For this review, take the finished solid that the model builds, in its own axes (mm). A direction names the side the tool comes from. Coordinates: 2 decimals unless noted, no trailing zeros. Loops run counter-clockwise (first coordinate to the right, second up) from the corner with the lowest first, then second, coordinate; pieces in that order, holes last. Notation, with made-up numbers: (58, -31.5) -> (81, -31.5) arc R6 ccw to (81, -26.5) -> close; hole circle Ø3 at (37.5, -36). An arc over 180 degrees is marked (long way). Use a Markdown table: item, result.
from build123d import *

# Parameters (mm, degrees)
F1_DEPTH     = 100
F0_R         = 2
F2_DEPTH     = 3
F3_DEPTH     = 40
F4_W         = 80
F4_H         = 60
F5_DEPTH     = 2
F7_DEPTH     = 25
F9_R         = 6
F10_T1_DEPTH = 40
F10_T3_DEPTH = 47.5
F11_R        = 0.99999
F12_SIZE     = 2.2


# Not quite as in the source:
# - a fillet or chamfer that OpenCascade refuses, or shapes differently, is made with other operations: its cross-section is extruded or revolved along the edge and cut away or added
# - a fillet or chamfer is up to 0.001 mm smaller than in the source, because OpenCascade refuses the exact size


with BuildPart() as f1:
    # F0 (on Right) → F1 (new body)
    with BuildSketch(Plane.YZ):
        Polygon((34.2351660257, -7.2769091786), (0, 0), (-34.2351660257, -7.2769091786), (-33.6114309532, -10.2113519808), (0, -3.0670217846), (33.6114309532, -10.2113519808), align=None)
    extrude(amount=F1_DEPTH)

    # F0 (on Right) → F2 (join)
    with BuildSketch(Plane.YZ):
        Polygon((5.3139140418, 25), (0, 0), (34.2351660257, -7.2769091786), (63.9481604091, 132.5117388406), (29.7129943835, 139.7886480192), align=None)
        with Locations((43.711902034, 121.4779794189)):
            Circle(F0_R, mode=Mode.SUBTRACT)
        Polygon((-5.3139140418, 25), (0, 0), (5.3139140418, 25), align=None)
        Polygon((-34.2351660257, -7.2769091786), (0, 0), (-5.3139140418, 25), (-29.7129943835, 139.7886480192), (-63.9481604091, 132.5117388406), align=None)
        with Locations((-43.711902034, 121.4779794189)):
            Circle(F0_R, mode=Mode.SUBTRACT)
    extrude(amount=F2_DEPTH)

    # F0 (on Right) → F3 (join)
    with BuildSketch(Plane.YZ):
        Polygon((-33.6114309532, -10.2113519808), (-34.2351660257, -7.2769091786), (-37.1696088279, -7.9006442511), (-38.209167282, -3.0099062474), (-40.1654624834, -3.425729629), (-38.5021689569, -11.2509104349), align=None)
        Polygon((37.1696088279, -7.9006442511), (34.2351660257, -7.2769091786), (33.6114309532, -10.2113519808), (38.5021689569, -11.2509104349), (40.1654624834, -3.425729629), (38.209167282, -3.0099062474), align=None)
    extrude(amount=F3_DEPTH)

    # F4 (on face) → F5 (join)
    with BuildSketch(Plane(origin=(0, 34.2351660257, -7.2769091786), x_dir=(-1, 0, 0), z_dir=(0, 0.9781476007, -0.2079116908))):
        Polygon((-3, 106.1880215352), (-83, 60), (-3, 60), align=None)
        with Locations((-43, 30)):
            Rectangle(F4_W, F4_H)
    extrude(amount=-F5_DEPTH)

    # F6 (on face) → F7 (cut)
    with BuildSketch(Plane(origin=(0, 34.2351660257, -7.2769091786), x_dir=(-1, 0, 0), z_dir=(0, 0.9781476007, -0.2079116908))):
        Polygon((-68.2907584126, 20.9817930688), (-37.1453792063, 3), (-6, 20.9817930688), (-6, 56.9453792063), (-37.1453792063, 74.927172275), (-68.2907584126, 56.9453792063), align=None)
    extrude(amount=-F7_DEPTH, mode=Mode.SUBTRACT)

    # F8: F1 across plane


with BuildPart() as f1_1:
    add(f1.part)
    add(f1.part.mirror(Plane.XZ))

    # F9
    f9_edges = [f1_1.edges().sort_by_distance(p)[0] for p in [
        (3, -55.33475, 96.798561),
        (3, 55.33475, 96.798561),
        (83, -45.73172, 51.619859),
        (83, 45.73172, 51.619859),
        (83, -33.257018, -7.068997),
        (83, 33.257018, -7.068997),
        (1.5, -5.313914, 25),
        (1.5, 5.313914, 25),
        (51.5, 0, 0),
        (50, 0, -3.067022),
        (1.5, -29.712994, 139.788648),
        (1.5, -63.94816, 132.511739),
        (1.5, 29.712994, 139.788648),
        (1.5, 63.94816, 132.511739),
    ]]
    fillet(f9_edges, radius=F9_R)

    # F10: fillet of radius 1.5 on 6 edges, made by hand

    # F10_s2 → F10_t1 (join)
    with BuildSketch(Plane.YZ):
        with BuildLine():
            ThreePointArc((34.5470335619, -5.8096877775), (34.7562491111, -6.9385138663), (35.7023874268, -7.5887767148))
            Line((35.7023874268, -7.5887767148), (34.2351660257, -7.2769091786))
            Line((34.2351660257, -7.2769091786), (34.5470335619, -5.8096877775))
        make_face()
        with BuildLine():
            ThreePointArc((35.7023874268, -7.5887767148), (36.8312135155, -7.3795611657), (37.4814763641, -6.43342285))
            Line((37.4814763641, -6.43342285), (37.1696088279, -7.9006442511))
            Line((37.1696088279, -7.9006442511), (35.7023874268, -7.5887767148))
        make_face()
        with BuildLine():
            ThreePointArc((-37.4814763641, -6.43342285), (-36.8312135155, -7.3795611657), (-35.7023874268, -7.5887767148))
            Line((-35.7023874268, -7.5887767148), (-37.1696088279, -7.9006442511))
            Line((-37.1696088279, -7.9006442511), (-37.4814763641, -6.43342285))
        make_face()
        with BuildLine():
            ThreePointArc((-34.5470335619, -5.8096877775), (-34.7562491111, -6.9385138663), (-35.7023874268, -7.5887767148))
            Line((-35.7023874268, -7.5887767148), (-34.2351660257, -7.2769091786))
            Line((-34.2351660257, -7.2769091786), (-34.5470335619, -5.8096877775))
        make_face()
    extrude(amount=F10_T1_DEPTH)

    # F10_s4 → F10_t3 (cut)
    with BuildSketch(Plane.YZ.offset(-3.75)):
        with BuildLine():
            ThreePointArc((-37.0349475558, -10.9390428987), (-38.1637736445, -10.7298273495), (-38.8140364931, -9.7836890338))
            Line((-38.8140364931, -9.7836890338), (-38.5021689569, -11.2509104349))
            Line((-38.5021689569, -11.2509104349), (-37.0349475558, -10.9390428987))
        make_face()
        with BuildLine():
            ThreePointArc((37.0349475558, -10.9390428987), (38.1637736445, -10.7298273495), (38.8140364931, -9.7836890338))
            Line((38.8140364931, -9.7836890338), (38.5021689569, -11.2509104349))
            Line((38.5021689569, -11.2509104349), (37.0349475558, -10.9390428987))
        make_face()
    extrude(amount=F10_T3_DEPTH, mode=Mode.SUBTRACT)

    # F11 (radius 1 in the source; OpenCascade refuses exactly that, so slightly less here)
    f11_edges = [f1_1.edges().sort_by_distance(p)[0] for p in [
        (20, 40.165462, -3.42573),
        (20, 38.209167, -3.009906),
        (20, -40.165462, -3.42573),
        (20, -38.209167, -3.009906),
    ]]
    fillet(f11_edges, radius=F11_R)

    # F12
    f12_edges = [f1_1.edges().sort_by_distance(p)[0] for p in [
        (3, -45.711902, 121.477979),
        (3, 41.711902, 121.477979),
    ]]
    chamfer(f12_edges, length=F12_SIZE)


solid = f1_1.part
(1) Take a section at A-A on z = 68.5. Write out the cut boundary in (x, y), plus the area to 3 significant figures.
Found:
| item | result |
|---|---|
| outline | (0, -50.34) -> (52.74, -50.34) -> (53.48, -48.3) -> (3, -48.3) -> (3, -14.56) -> (0, -14.56) -> close; (0, 14.56) -> (3, 14.56) -> (3, 48.3) -> (53.48, 48.3) -> (52.74, 50.34) -> (0, 50.34) -> close |
| area | 420 mm^2 |
(2) Mouldability with a two-part tool opening along Y and no side actions: class faces 1 (the face through (19.72, 39.38, -7.13)), 2 (the face through (19.72, -39.394, -7.056)), 3 (the face through (52.571, 46.264, 58.934)) as pulls with the +Y half, pulls with the -Y half, needs draft (parallel to the pull), parting line crosses it, or undercut.
Found:
| item | result |
|---|---|
| face 1 | pulls with the +Y half |
| face 2 | pulls with the -Y half |
| face 3 | undercut |
(3) Take a section at C-C on x = 91. Write out the cut boundary in (y, z).
Found:
| item | result |
|---|---|
| outline | (-34.24, -7.28) -> (-33.61, -10.21) -> (-1.25, -3.33) arc R6 cw to (1.25, -3.33) -> (33.61, -10.21) -> (34.24, -7.28) -> (1.25, -0.27) arc R6 ccw to (-1.25, -0.27) -> close |
(4) Take a section at B-B on x = 48. Write out the cut boundary in (y, z), plus the area to 3 significant figures.
Found:
| item | result |
|---|---|
| outline | (-50.91, 71.18) -> (-48.51, 59.88) -> (-46.55, 60.3) -> (-48.95, 71.59) -> close; (-36.16, 1.79) -> (-33.61, -10.21) -> (-1.25, -3.33) arc R6 cw to (1.25, -3.33) -> (33.61, -10.21) -> (36.16, 1.79) -> (34.21, 2.2) -> (32.28, -6.86) -> (1.25, -0.27) arc R6 ccw to (-1.25, -0.27) -> (-32.28, -6.86) -> (-34.21, 2.2) -> close; (46.55, 60.3) -> (48.51, 59.88) -> (50.91, 71.18) -> (48.95, 71.59) -> close |
| area | 291 mm^2 |
(5) For line 1 along X through (y, z) = (38, 18); line 2 along X through (y, z) = (-19.5, 5); line 3 along Y through (x, z) = (68.5, 35), list the stretches that pass through material, from the lowest coordinate up.
Found:
| item | result |
|---|---|
| line 1 | x = 0 to 6, 68.29 to 83 |
| line 2 | x = 0 to 3 |
| line 3 | y = -43.22 to -41.18, 41.18 to 43.22 |
(6) Take a section at D-D on y = 25.5. Write out the cut boundary in (x, z), plus the area to 3 significant figures.
Found:
| item | result |
|---|---|
| outline | (0, -8.49) -> (100, -8.49) -> (100, -5.42) -> (3, -5.42) -> (3, 119.97) -> (0, 119.97) -> close |
| area | 683 mm^2 |
(7) For pin 1 Ø5 at (y, z) = (43.71, 121.48) entering from +X; pin 2 Ø2 at (x, z) = (16, 69) entering from +Y; pin 3 Ø0.7 at (x, y) = (1.5, 0) entering from +Z, all flat-tipped, find the tip position at first contact; note any pin that passes through.
Found:
| item | result |
|---|---|
| pin 1 | stops at x = 1.3 |
| pin 2 | stops at y = 50.66 |
| pin 3 | stops at z = 25 |
(8) For faces 4 (the face through (40, -38, -8)), 5 (the face through (52.571, -46.264, 58.934)), 6 (the face through (68.291, -41, 31)), 7 (the face through (52.5, 47.006, 57.547)), list the 3-axis set-ups (+Z, -Z, +X, -X, +Y, -Y) from which the entire face can be reached by the end or side of a thin tool; tool diameter is ignored.
Found:
| item | result |
|---|---|
| face 4 | -Z, +X, -Y |
| face 5 | +Z, +X |
| face 6 | +Y, -Y |
| face 7 | -Z |
